Input: dimensioned drawing with shaded views. Units: mm. Origin: part minimum x, y, z. A direction names the side the tool comes from. Give positions to 0.01 mm unless a question says otherwise; leave off trailing zeros. Loops run counter-clockwise (first coordinate to the right, second up) from the corner with the lowest first, then second, coordinate; pieces in that order, holes last. Notation, with made-up numbers: M 32.25,11.5 L 73.25,11.5 A29 ccw 73.25,44.5 Z; hole C 85,-10 d11. An arc over 180 degrees is marked long. Answer in a Markdown table with one row per item.
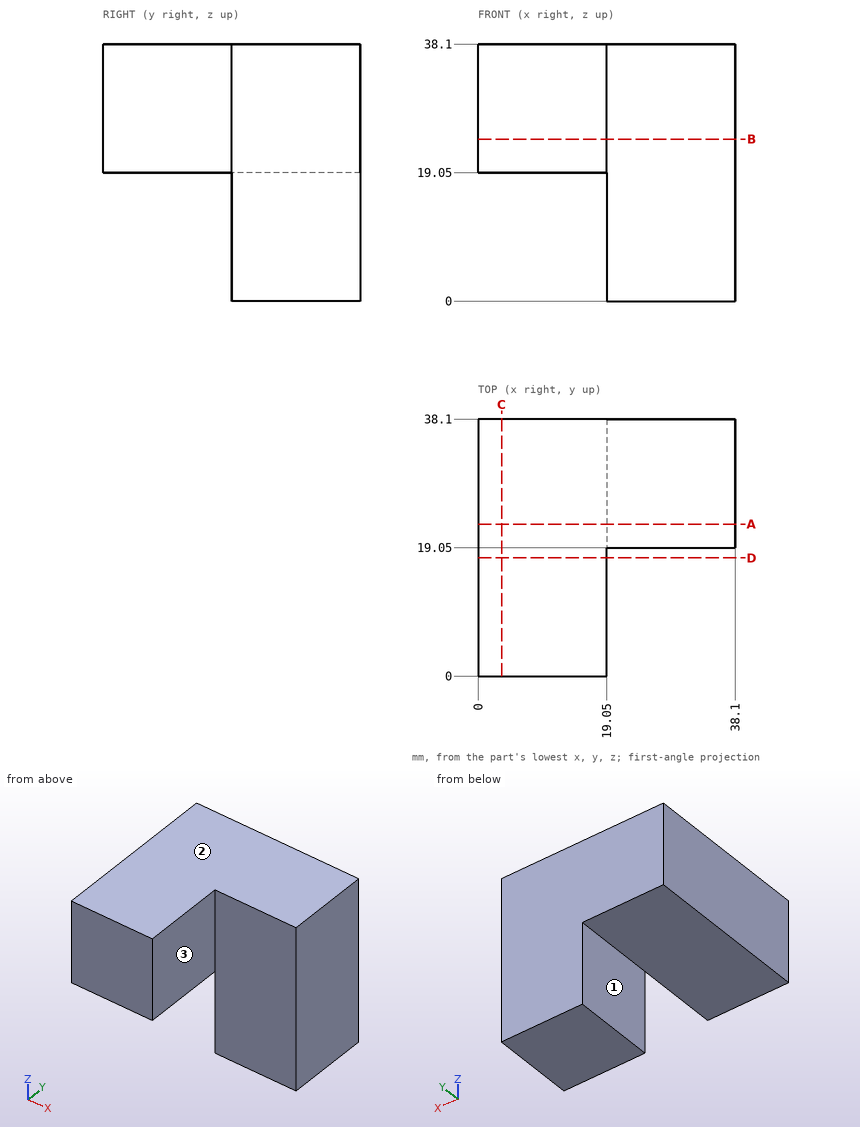
Q1. Section query D-D (y = 17.5). Output: boundary loops of the cut face in (x, z).
Values follow:
| item | result |
|---|---|
| outline | M 0,19.05 L 19.05,19.05 L 19.05,38.1 L 0,38.1 Z |
Q2. Ray query, probe 1 along Z at (x, y) = (8.5, 2); probe 2 along X at (y, z) = (5, 29.5). Return the intervals inside material, ascending. Write a range as from..to.
Values follow:
| item | result |
|---|---|
| probe 1 | 19.05..38.1 |
| probe 2 | 0..19.05 |
Q3. Reachability of the marked faces 1, 2 and 3 from +Z, -Z, +X, -X, +Y, -Y: full face, straight path, thin tool, end or side. Return the list, or none.
Values follow:
| item | result |
|---|---|
| face 1 | -Z, -X, +Y, -Y |
| face 2 | +Z, +X, -X, +Y, -Y |
| face 3 | +Z, -Z, +X, -Y |
Q4. Section query B-B (z = 24). Output: boundary loops of the cut face in (x, y).
Values follow:
| item | result |
|---|---|
| outline | M 0,0 L 19.05,0 L 19.05,19.05 L 38.1,19.05 L 38.1,38.1 L 0,38.1 Z |
Q5. Contact query for flat-ended pins moving along their axis: pin 1 Ø9.5 at (y, z) = (6.5, 26.5) entering from +X; pin 2 Ø8 at (x, z) = (28.5, 13) entering from -Y; pin 3 Ø4 at (y, z) = (18.5, 11) entering from +X; pin 4 Ø15 at (y, z) = (33, 6) entering from -X. Output: stop coordinate, or through.
Values follow:
| item | result |
|---|---|
| pin 1 | x = 19.05 |
| pin 2 | y = 19.05 |
| pin 3 | x = 38.1 |
| pin 4 | x = 19.05 |
Q6. Section query C-C (x = 3.5). Output: boundary loops of the cut face in (y, z).
Values follow:
| item | result |
|---|---|
| outline | M 0,19.05 L 38.1,19.05 L 38.1,38.1 L 0,38.1 Z |
Q7. Section query A-A (y = 22.5). Output: boundary loops of the cut face in (x, z).
Values follow:
| item | result |
|---|---|
| outline | M 0,19.05 L 19.05,19.05 L 19.05,0 L 38.1,0 L 38.1,38.1 L 0,38.1 Z |
